```python
from build123d import *

# Parameters (mm, degrees)
CROQUIS1_W                 = 20
CROQUIS1_H                 = 20
SALIENTE_EXTRUIR1_DEPTH    = 30
CORTAR_EXTRUIR1_DEPTH      = 37.007356213
CORTAR_EXTRUIR1_DEPTH_BACK = 37.007356213
CROQUIS4_R                 = 1.5875
CORTAR_EXTRUIR2_DEPTH      = 30
CROQUIS7_R                 = 3.175
SALIENTE_EXTRUIR2_DEPTH    = 20
CORTAR_EXTRUIR3_DEPTH      = 39.627579186


with BuildPart() as part:
    # Croquis1 → Saliente-Extruir1 (new body)
    with BuildSketch(Plane(origin=(0, 0, 0), x_dir=(1, 0, 0), z_dir=(0, 1, 0))):
        with Locations((3.859649123, 4.298245614)):
            Rectangle(CROQUIS1_W, CROQUIS1_H)
    extrude(amount=SALIENTE_EXTRUIR1_DEPTH)

    # Croquis2 → Cortar-Extruir1 (cut, two sides: drawn at the far end of the back side and taken through both)
    with BuildSketch(Plane.XY.offset(-CORTAR_EXTRUIR1_DEPTH_BACK)):
        Polygon((13.859649123, 24.692447492), (13.859649123, 18.444349321), (11.150769621, 23.124565022), align=None)
    extrude(amount=CORTAR_EXTRUIR1_DEPTH + CORTAR_EXTRUIR1_DEPTH_BACK, mode=Mode.SUBTRACT)

    # Croquis4 → Cortar-Extruir2 (cut)
    with BuildSketch(Plane(origin=(18.37833915, 10.637267462, 0), x_dir=(0, 0, -1), z_dir=(0.8654839376667617, 0.5009366762783868, 0))):
        with Locations(Location((4.298245614, 11.724295816, 0), (0, 0, 90))):
            Circle(CROQUIS4_R)
    extrude(amount=-CORTAR_EXTRUIR2_DEPTH, mode=Mode.SUBTRACT)

    # Croquis7 → Saliente-Extruir2 (add)
    with BuildSketch(Plane.XZ):
        with Locations(Location((3.859649123, -4.298245614, 0), (0, 0, 270))):
            Circle(CROQUIS7_R)
    extrude(amount=SALIENTE_EXTRUIR2_DEPTH)

    # Croquis9 → Cortar-Extruir3 (cut, through all)
    with BuildSketch(Plane.XY.offset(5.701754386)):
        Polygon((10.065279616, 25), (-6.140350877, 25), (-6.140350877, 30), (13.859649123, 30), (13.859649123, 18.444349321), align=None)
    extrude(amount=-CORTAR_EXTRUIR3_DEPTH, mode=Mode.SUBTRACT)


solid = part.part
```
Could you check a few things on this model? Use its own coordinates, in mm. A direction names the side the tool comes from. Round coordinates to 2 decimals unless told otherwise and drop trailing zeros. Write each loop counter-clockwise with the first axis right and the second up, starting at its lowest first coordinate (ties: lowest second). Pieces come first, ordered by that corner, then holes. Notation, with made-up numbers: M 87,57.25 L 139,57.25 A14 ccw 139,82.25 Z; hole C 23,75 d2. An arc over 180 degrees is marked long. Answer in a Markdown table with one row per item. Add a question column.
Q1. If I drill on line 1 (Z direction, x = 3.75, y = -1.5); line 2 (Y direction, x = 0.75, z = -12.25); line 3 (X direction, y = 23.5, z = -12.5), over which ranges is the centre line in solid material (lowest first)? Write a range as from..to.
Q2. Imagine slicing it at A-A (z = -10). Please give me the cut outline in (x, y).
Q3. Imagine slicing it at B-B (y = -11). Please give me the cut outline in (x, z) (3 decimals), then the cut area to 3 significant figures.
Q4. On a 3-axis mill with a long thin cutter (end or side, diameter ignored), from which of +Z, -Z, +X, -X, +Y, -Y can I reach the whole of each face in a straight line? I mean faces 5 (the cylindrical face through (1.04, -9.86, -5.76)), 6 (the flat face through (4, 12, -14.298)). Say none if no direction works.
Q5. Will these pins go through, and if not, where does the flat tip stop? pin 1 Ø5 at (y, z) = (-5.5, -9.5) entering from +X; pin 2 Ø5 at (x, z) = (10.5, -10) entering from -Y; pin 3 Ø1 at (x, y) = (5.5, -12.5) entering from +Z.
Q6. If we mould it in two halves opening along Y, with no side actions, what happens to faces 1 (the flat face through (4, 12, 5.702)), 2 (the flat face through (2, 25, -4)), 3 (the flat face through (4, -20, -4)), 4 (the cylindrical face through (3.678, 13.843, -4.228))? For each: +Y half, -Y half, draft (parallel to the pull), parting line (faces both ways), or undercut.
Values:
| question | item | result |
|---|---|---|
| 1 | line 1 | -7.47..-1.13 |
| 1 | line 2 | 0..25 |
| 1 | line 3 | -6.14..10.93 |
| 2 | outline | M -6.14,0 L 13.86,0 L 13.86,18.44 L 10.07,25 L -6.14,25 Z |
| 3 | outline | C 3.86,-4.298 d6.35 |
| 3 | area | 31.7 mm^2 |
| 4 | face 5 | -Y |
| 4 | face 6 | -Z, +X, -X, +Y, -Y |
| 5 | pin 1 | x = 5.53 |
| 5 | pin 2 | y = 0 |
| 5 | pin 3 | z = -1.34 |
| 6 | face 1 | draft |
| 6 | face 2 | +Y half |
| 6 | face 3 | -Y half |
| 6 | face 4 | undercut |
